Build history of the part. All positions in model axes, mm. A direction names the side the tool comes from. Give positions to 0.01 mm unless a question says otherwise; leave off trailing zeros. Order: outer loops, then holes, each group sorted by start corner. A loop starts at its lowest first (then second) coordinate and runs counter-clockwise, first axis right, second up. Notation, with made-up numbers: (67, 24) - (99, 24) arc R25 ccw to (99, 37) - close; hole circle Ø1 at (3.5, 71.25). An arc over 180 degrees is marked (long way). Use a Markdown table: item, result. Add a question column.
(1) Mould opens along X. For faces 3 (the face through (69, 0.1, 2)), 4 (the face through (40.56, 18.34, 2.46)), 5 (the face through (0, 11, 2)) say: +X half, -X half, draft (parallel to the pull), parting line (faces both ways), or undercut.
(2) Slice it at B-B (z = 1.9). Count the separate pieces of the cut face and the enclosed holes in it, then the cut area to 3 significant figures.
(3) Slice it at A-A (x = 50). Write the cut outline in (y, z).
(4) Wall check: line 1 (Y direction, x = 130.5, z = 2.4); line 2 (X direction, y = 20, z = 4.15); line 3 (Y direction, x = 132, z = 3.5). Give the ranges that are in metal, low to high.
(5) Which spindle directions (+Z, -Z, +X, -X, +Y, -Y) get a long thin tool onto all of the face, cutting with end or side? Do faces 1 (the face through (140, 11, 2)), 2 (the face through (31.5, 10, 2)). Say none if no direction does.
from build123d import *

# Parameters (mm, degrees)
SKETCH_1_R      = 3
EXTRUDE_1_DEPTH = 5


with BuildPart() as part:
    # 스케치1 → 보스-돌출1 (new body)
    with BuildSketch(Plane.XY):
        Polygon((0, 22.1), (0, 10.1), (0, 0.1), (140, 0.1), (140, 10.1), (140, 22.1), align=None)
        with BuildLine():
            Line((31.428932188, 2.528932188), (31.428932188, 3.028932188))
            Line((31.428932188, 3.028932188), (31.428932188, 3.528932188))
            ThreePointArc((31.428932188, 3.528932188), (32.928932188, 5.028932188), (34.428932188, 3.528932188))
            Line((34.428932188, 3.528932188), (34.428932188, 3.028932188))
            Line((34.428932188, 3.028932188), (34.428932188, 2.528932188))
            ThreePointArc((34.428932188, 2.528932188), (32.928932188, 1.028932188), (31.428932188, 2.528932188))
        make_face(mode=Mode.SUBTRACT)
        with BuildLine():
            Line((48.571067812, 3.528932188), (48.571067812, 3.028932188))
            Line((48.571067812, 3.028932188), (48.571067812, 2.528932188))
            ThreePointArc((48.571067812, 2.528932188), (47.071067812, 1.028932188), (45.571067812, 2.528932188))
            Line((45.571067812, 2.528932188), (45.571067812, 3.028932188))
            Line((45.571067812, 3.028932188), (45.571067812, 3.528932188))
            ThreePointArc((45.571067812, 3.528932188), (47.071067812, 5.028932188), (48.571067812, 3.528932188))
        make_face(mode=Mode.SUBTRACT)
        with BuildLine():
            ThreePointArc((12.5, 10.1), (9.5, 7.1), (6.5, 10.1))
            ThreePointArc((6.5, 10.1), (9.5, 13.1), (12.5, 10.1))
        make_face(mode=Mode.SUBTRACT)
        with BuildLine():
            Line((28.5, 8.6), (28.5, 10.1))
            Line((28.5, 10.1), (28.5, 11.6))
            ThreePointArc((28.5, 11.6), (30, 13.1), (31.5, 11.6))
            Line((31.5, 11.6), (31.5, 10.1))
            Line((31.5, 10.1), (31.5, 8.6))
            ThreePointArc((31.5, 8.6), (30, 7.1), (28.5, 8.6))
        make_face(mode=Mode.SUBTRACT)
        with BuildLine():
            Line((32.5, 9.6), (32.5, 10.1))
            Line((32.5, 10.1), (32.5, 10.6))
            ThreePointArc((32.5, 10.6), (34.696699141, 15.903300859), (40, 18.1))
            ThreePointArc((40, 18.1), (45.303300859, 15.903300859), (47.5, 10.6))
            Line((47.5, 10.6), (47.5, 10.1))
            Line((47.5, 10.1), (47.5, 9.6))
            ThreePointArc((47.5, 9.6), (40, 2.1), (32.5, 9.6))
        make_face(mode=Mode.SUBTRACT)
        with BuildLine():
            Line((51.5, 11.6), (51.5, 10.1))
            Line((51.5, 10.1), (51.5, 8.6))
            ThreePointArc((51.5, 8.6), (50, 7.1), (48.5, 8.6))
            Line((48.5, 8.6), (48.5, 10.1))
            Line((48.5, 10.1), (48.5, 11.6))
            ThreePointArc((48.5, 11.6), (50, 13.1), (51.5, 11.6))
        make_face(mode=Mode.SUBTRACT)
        with Locations((70.5, 10.1)):
            Circle(SKETCH_1_R, mode=Mode.SUBTRACT)
        with Locations((100.5, 10.1)):
            Circle(SKETCH_1_R, mode=Mode.SUBTRACT)
        with Locations((130.5, 10.1)):
            Circle(SKETCH_1_R, mode=Mode.SUBTRACT)
        with BuildLine():
            Line((31.428932188, 16.671067812), (31.428932188, 17.171067812))
            Line((31.428932188, 17.171067812), (31.428932188, 17.671067812))
            ThreePointArc((31.428932188, 17.671067812), (32.928932188, 19.171067812), (34.428932188, 17.671067812))
            Line((34.428932188, 17.671067812), (34.428932188, 17.171067812))
            Line((34.428932188, 17.171067812), (34.428932188, 16.671067812))
            ThreePointArc((34.428932188, 16.671067812), (32.928932188, 15.171067812), (31.428932188, 16.671067812))
        make_face(mode=Mode.SUBTRACT)
        with BuildLine():
            Line((45.571067812, 16.671067812), (45.571067812, 17.171067812))
            Line((45.571067812, 17.171067812), (45.571067812, 17.671067812))
            ThreePointArc((45.571067812, 17.671067812), (47.071067812, 19.171067812), (48.571067812, 17.671067812))
            Line((48.571067812, 17.671067812), (48.571067812, 17.171067812))
            Line((48.571067812, 17.171067812), (48.571067812, 16.671067812))
            ThreePointArc((48.571067812, 16.671067812), (47.071067812, 15.171067812), (45.571067812, 16.671067812))
        make_face(mode=Mode.SUBTRACT)
        with BuildLine():
            Line((38.5, 19.8), (38.5, 20.1))
            Line((38.5, 20.1), (38.5, 20.4))
            ThreePointArc((38.5, 20.4), (40, 21.967353054), (41.5, 20.4))
            Line((41.5, 20.4), (41.5, 20.1))
            Line((41.5, 20.1), (41.5, 19.8))
            ThreePointArc((41.5, 19.8), (40, 18.232646946), (38.5, 19.8))
        make_face(mode=Mode.SUBTRACT)
    extrude(amount=EXTRUDE_1_DEPTH)


solid = part.part
Solution:
| question | item | result |
|---|---|---|
| 1 | face 3 | draft |
| 1 | face 4 | undercut |
| 1 | face 5 | -X half |
| 2 | separate pieces | 1 |
| 2 | enclosed holes | 12 |
| 2 | area | 2,690 mm2 |
| 3 | outline | (0.1, 0) - (7.1, 0) - (7.1, 5) - (0.1, 5) - close; (13.1, 0) - (22.1, 0) - (22.1, 5) - (13.1, 5) - close |
| 4 | line 1 | 0.1 to 7.1, 13.1 to 22.1 |
| 4 | line 2 | 0 to 38.5, 41.5 to 140 |
| 4 | line 3 | 0.1 to 7.5, 12.7 to 22.1 |
| 5 | face 1 | +Z, -Z, +X, +Y, -Y |
| 5 | face 2 | +Z, -Z |
